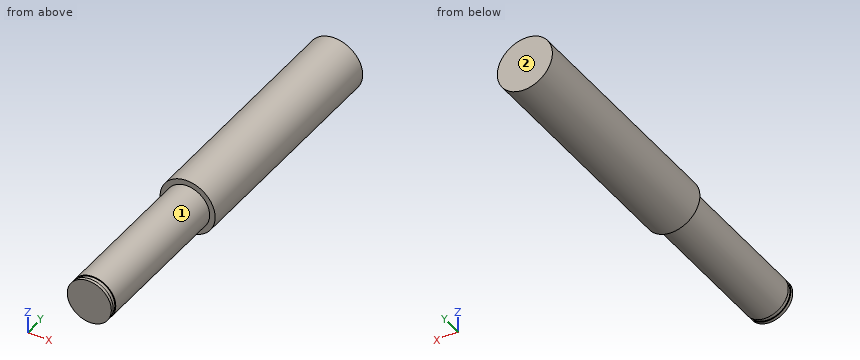
from build123d import *

# Parameters (mm, degrees)
F0_R     = 7.5
F1_DEPTH = 105
F2_R     = 7.5
F2_R_2   = 6
F3_DEPTH = 42
F5_R     = 6
F5_R_2   = 5.75
F6_DEPTH = 1.1


with BuildPart() as f1:
    # F0 (on Front) → F1 (new body)
    with BuildSketch(Plane.XZ):
        Circle(F0_R)
    extrude(amount=F1_DEPTH)

    # F2 (on face) → F3 (cut)
    with BuildSketch(Plane.XZ.offset(105)):
        Circle(F2_R)
        Circle(F2_R_2, mode=Mode.SUBTRACT)
    extrude(amount=-F3_DEPTH, mode=Mode.SUBTRACT)

    # F5 (on offset) → F6 (cut)
    with BuildSketch(Plane.XZ.offset(104.2)):
        Circle(F5_R)
        Circle(F5_R_2, mode=Mode.SUBTRACT)
    extrude(amount=-F6_DEPTH, mode=Mode.SUBTRACT)


solid = f1.part
Here's how the part is built. I have some questions about the finished solid (model axes, mm). Face numbers are marked on the shaded views. A direction names the side the tool comes from. Coordinates: 2 decimals unless noted, no trailing zeros. Loops run counter-clockwise (first coordinate to the right, second up) from the corner with the lowest first, then second, coordinate; pieces in that order, holes last.
1. Imagine slicing it at A-A, the plane x = 0. Please give me the cut outline in (y, z), and give its area (3 significant figures).
2. Imagine slicing it at D-D, the plane y = -35. Please give me the cut outline in (x, z), and give its area (3 significant figures).
3. For P1, Ø1.5, axis at y = -82, z = 4.5, coming from the -X side; P2, Ø4, axis at x = -6, y = -87.5, coming from the -Z side; P3, Ø2, axis at y = -51.5, z = 3, coming from the -X side, each with a flat end and sliding along its axis, tell me the tip position at first contact or that it passes through.
4. I need wall thicknesses on L1, parallel to Z at x = -0.5, y = -56; L2, parallel to X at y = -38, z = 4.5. Which ranges of each line are inside material? Lowest first, please.
5. Imagine slicing it at B-B, the plane z = 0. Please give me the cut outline in (x, y).
6. Imagine slicing it at C-C, the plane y = -79.5. Please give me the cut outline in (x, z), and give its area (3 significant figures).
7. For the marked faces 1 and 2, which set-ups out of +Z, -Z, +X, -X, +Y, -Y let a thin tool reach every point of the face, with its end or its side?
Taken from the geometry:
1. outline: (-105, -6) - (-104.2, -6) - (-104.2, -5.75) - (-103.1, -5.75) - (-103.1, -6) - (-63, -6) - (-63, -7.5) - (0, -7.5) - (0, 7.5) - (-63, 7.5) - (-63, 6) - (-103.1, 6) - (-103.1, 5.75) - (-104.2, 5.75) - (-104.2, 6) - (-105, 6) - close
1. area: 1,450 mm2
2. outline: circle Ø15 at (0, 0)
2. area: 177 mm2
3. P1: stops at x = -4.68
3. P2: stops at z = -4.47
3. P3: stops at x = -7.23
4. L1: z = -7.48 to 7.48
4. L2: x = -6 to 6
5. outline: (-7.5, -63) - (-6, -63) - (-6, -103.1) - (-5.75, -103.1) - (-5.75, -104.2) - (-6, -104.2) - (-6, -105) - (6, -105) - (6, -104.2) - (5.75, -104.2) - (5.75, -103.1) - (6, -103.1) - (6, -63) - (7.5, -63) - (7.5, 0) - (-7.5, 0) - close
6. outline: circle Ø12 at (0, 0)
6. area: 113 mm2
7. face 1: -Y
7. face 2: +Z, -Z, +X, -X, +Y
